from build123d import *

# Parameters (mm, degrees)
BOSS_EXTRUDE1_DEPTH = 2
BOSS_EXTRUDE2_START = 2
SKETCH2_R           = 7.25
BOSS_EXTRUDE2_DEPTH = 2
BOSS_EXTRUDE3_DEPTH = 3
SKETCH4_R           = 2.75
CUT_EXTRUDE1_DEPTH  = 22.427202337
SKETCH5_R           = 4
CUT_EXTRUDE2_DEPTH  = 1
SKETCH6_R           = 1.5
CUT_EXTRUDE3_DEPTH  = 22.728437588
FILLET1_R           = 10
CUT_EXTRUDE4_DEPTH  = 18


with BuildPart() as part:
    # Sketch1 → Boss-Extrude1 (new, symmetric)
    with BuildSketch(Plane(origin=(0, 0, 0), x_dir=(1, 0, 0), z_dir=(0, 1, 0))):
        with BuildLine():
            Line((-4, -5.953306689), (-4, 12))
            ThreePointArc((-4, 12), (0, 16), (4, 12))
            Line((4, 12), (4, -5.953306689))
            ThreePointArc((4, -5.953306689), (0, -19.25), (-4, -5.953306689))
        make_face()
    extrude(amount=BOSS_EXTRUDE1_DEPTH, both=True)

    # Sketch2 → Boss-Extrude2 (add)
    with BuildSketch(Plane(origin=(0, 2, 0), x_dir=(1, 0, 0), z_dir=(0, 1, 0)).offset(BOSS_EXTRUDE2_START)):
        with Locations(Location((0, -12, 0), (0, 0, 56.514623377))):
            Circle(SKETCH2_R)
    extrude(amount=-BOSS_EXTRUDE2_DEPTH)

    # Sketch3 → Boss-Extrude3 (add)
    with BuildSketch(Plane(origin=(0, 2, 0), x_dir=(1, 0, 0), z_dir=(0, 1, 0))):
        with BuildLine():
            Line((-3, 12), (-3, 8))
            ThreePointArc((-3, 8), (0, 5), (3, 8))
            Line((3, 8), (3, 12))
            ThreePointArc((3, 12), (0, 15), (-3, 12))
        make_face()
    extrude(amount=BOSS_EXTRUDE3_DEPTH)

    # Sketch4 → Cut-Extrude1 (cut, through all)
    with BuildSketch(Plane(origin=(0, 4, 0), x_dir=(1, 0, 0), z_dir=(0, 1, 0))):
        with Locations(Location((0, -12, 0), (0, 0, 270))):
            Circle(SKETCH4_R)
    extrude(amount=-CUT_EXTRUDE1_DEPTH, mode=Mode.SUBTRACT)

    # Sketch5 → Cut-Extrude2 (cut)
    with BuildSketch(Plane.XZ.offset(2)):
        with Locations(Location((0, 12, 0), (0, 0, 270))):
            Circle(SKETCH5_R)
    extrude(amount=-CUT_EXTRUDE2_DEPTH, mode=Mode.SUBTRACT)

    # Sketch6 → Cut-Extrude3 (cut, through all)
    with BuildSketch(Plane.XZ.offset(2)):
        with Locations(Location((0, -12, 0), (0, 0, 270))):
            Circle(SKETCH6_R)
        with Locations(Location((0, -8, 0), (0, 0, 270))):
            Circle(SKETCH6_R)
        with Locations(Location((0, 3, 0), (0, 0, 270))):
            Circle(SKETCH6_R)
    extrude(amount=-CUT_EXTRUDE3_DEPTH, mode=Mode.SUBTRACT)

    # Fillet1
    fillet1_edges = [part.edges().sort_by_distance(p)[0] for p in [
        (-4, 0, 5.953306689),
        (4, 0, 5.953306689),
    ]]
    fillet(fillet1_edges, radius=FILLET1_R)

    # Sketch7 → Cut-Extrude4 (cut)
    with BuildSketch(Plane.XY):
        Polygon((-7.25, -2), (-5.75, -2), (-7.25, -0.5), align=None)
        Polygon((7.25, -2), (5.75, -2), (7.25, -0.5), align=None)
    extrude(amount=CUT_EXTRUDE4_DEPTH, mode=Mode.SUBTRACT)


solid = part.part
Model file for the job. Use its own axes, mm. A direction names the side the tool comes from. Coordinates: 2 decimals unless noted, no trailing zeros. Order: outer loops, then holes, each group sorted by start corner. A loop starts at its lowest first (then second) coordinate and runs counter-clockwise, first axis right, second up. Notation, with made-up numbers: (-30, 8.5) -> (5, 8.5) arc R15 cw to (5, 18.5) -> close; hole circle Ø1 at (53.25, 30). An arc over 180 degrees is marked (long way). Return JSON: item names as keys, results as strings. Group by question number.
Item 1: Saw through at D-D on z = -10. Write the cut outline in (x, y), then the cut area to 3 significant figures.
Item 2: Saw through at B-B on y = 1.5. Write the cut outline in (x, z).
Item 3: Flat gauge pins, fed straight in: P1, Ø1.5, axis at y = 4, z = -10.5, coming from the -X side; P2, Ø1.5, axis at x = -0.5, z = -0.5, coming from the +Y side; P3, Ø4, axis at x = -3.5, y = 2, coming from the +Z side; P4, Ø2.5, axis at x = 0, z = 3, coming from the +Y side. Where does each tip first touch, or does it go through?
Item 4: Tool access for faces 1 (the cylindrical face through (0, 3, -15)), 2 (the flat face through (3, 4, 14)), 3 (the cylindrical face through (0, 3, -5)), 4 (the flat face through (-3, 3, -10)): list every direction of +Z, -Z, +X, -X, +Y, -Y with a clear straight run to the whole face (end or side of a thin tool).
Item 5: Saw through at A-A on z = 12. Write the cut outline in (x, y).
Item 6: Wall check: line 1 along X through (y, z) = (3, 12); line 2 along Y through (x, z) = (-2.5, 4); line 3 along X through (y, z) = (1, 9.5). Give the ranges that are in metal, low to high. Write a range as [from, to].
Item 7: Pull direction Z, two halves, no side cores. Call faces 5 (the flat face through (6.32, -1.43, 11.93)), 6 (the cylindrical face through (-4.496, 0.028, 5.033)), 7 (the flat face through (-3, -1, 13)): pulls with the +Z half, pulls with the -Z half, needs draft (parallel to the pull), parting line crosses it, or undercut.
Item 8: Saw through at C-C on y = 3. Write the cut outline in (x, z).
Values found:
{
 "1": {"outline": "(-4, -2) -> (4, -2) -> (4, 2) -> (3, 2) -> (3, 5) -> (-3, 5) -> (-3, 2) -> (-4, 2) -> close", "area": "50.0 mm2"},
 "2": {"outline": "(-5.88, 7.76) arc R10 cw to (-4, 1.92) -> (-4, -12) arc R4 ccw to (4, -12) -> (4, 1.92) arc R10 cw to (5.88, 7.76) arc R7.25 ccw (long way) to start; hole circle Ø5.5 at (0, 12); hole circle Ø3 at (0, -12); hole circle Ø3 at (0, -8); hole circle Ø3 at (0, 3)"},
 "3": {"P1": "stops at x = -3", "P2": "stops at y = 2", "P3": "stops at z = 19.09", "P4": "passes through"},
 "4": {"face 1": "-Z, +Y", "face 2": "+Z, +X, -X, +Y", "face 3": "+Y", "face 4": "-Z, -X, +Y"},
 "5": {"outline": "(-7.25, -0.5) -> (-5.75, -2) -> (-4, -2) -> (-4, -1) -> (-2.75, -1) -> (-2.75, 4) -> (-7.25, 4) -> close; (2.75, -1) -> (4, -1) -> (4, -2) -> (5.75, -2) -> (7.25, -0.5) -> (7.25, 4) -> (2.75, 4) -> close"},
 "6": {"line 1": "x = [-7.25, -2.75], [2.75, 7.25]", "line 2": "y = [-2, 2]", "line 3": "x = [-6.81, -1.15], [1.15, 6.81]"},
 "7": {"face 5": "needs draft", "face 6": "pulls with the -Z half", "face 7": "undercut"},
 "8": {"outline": "circle Ø14.5 at (0, 12); (-3, -12) arc R3 ccw to (3, -12) -> (3, -8) arc R3 ccw to (-3, -8) -> close; hole circle Ø5.5 at (0, 12); hole circle Ø3 at (0, -12); hole circle Ø3 at (0, -8)"}
}
